Autodesk Inventor part; units mm, degrees
ref_plane "YZ Plane" through (0, 0, 0) normal (1, 0, 0) x (0, 1, 0)
ref_plane "XZ Plane" through (0, 0, 0) normal (0, 1, 0) x (-1, 0, 0)
ref_plane "XY Plane" through (0, 0, 0) normal (0, 0, 1) x (1, 0, 0)
sketch "Skizze1" plane through (0, 0, 0) normal (0, 0, 1) x (1, 0, 0)
  line L0 (-65.8319, 0) -> (313.5681, 0)
  line L1 (0, -176.4249) -> (0, 176.4249)
  line L2 (13.3681, -123) -> (13.3681, 123)
  line L3 (13.3681, -125.5) -> (259.3681, -125.5) construction
  line L4 (10.8681, 125.5) -> (-11.6319, 125.5)
  line L5 (-11.6319, 125.5) -> (-11.6319, 104.5)
  line L6 (10.8681, -125.5) -> (-11.6319, -125.5)
  line L7 (13.3681, -125.5) -> (35.8681, -125.5) construction
  line L8 (-11.6319, -125.5) -> (-11.6319, -124)
  line L9 (-11.6319, -124) -> (10.8681, -124)
  line L10 (11.8681, -123) -> (11.8681, 123)
  line L11 (10.8681, 124) -> (-10.1319, 124)
  line L12 (-10.1319, 124) -> (-10.1319, 104.5)
  line L13 (-10.1319, 104.5) -> (-11.6319, 104.5)
  arc A0 (13.3681, 123) -> (10.8681, 125.5) centre (10.8681, 123) ccw
  arc A1 (10.8681, -125.5) -> (13.3681, -123) centre (10.8681, -123) ccw
  arc A2 (10.8681, -124) -> (11.8681, -123) centre (10.8681, -123) ccw
  arc A3 (11.8681, 123) -> (10.8681, 124) centre (10.8681, 123) ccw
  point P0 (0, 0)
  point P1 (13.3681, 125.5)
  point P2 (11.8681, -124)
  point P3 (11.8681, 124)
  dimension "d0" = 251
  dimension "d1" = 90
  dimension "d2" = 25
  dimension "d3" = 90
  dimension "d4" = 21
  dimension "d5" = 90
  dimension "d6" = 25
  dimension "d7" = 180
  dimension "d8" = 1.5
  dimension "d9" = 90
  dimension "d10" = 23.5
  dimension "d11" = 90
  dimension "d12" = 248
  dimension "d13" = 90
  dimension "d14" = 22
  dimension "d15" = 90
  dimension "d17" = 1
extrude "Extrusion1" add sketch "Skizze1" along normal mid plane 193 contours L10 A3 L11 L1 L4 A0 L2 L0 | L0 L2 A1 L6 L1 L9 A2 L10 | L1 L6 L8 L9 | L11 L12 L13 L5 L4 L1
sketch "Skizze2" plane through (-11.6319, 104.5, 96.5) normal (-1, 0, 0) x (0, 0, 1)
  line L0 (-96.5, -280.2) -> (-96.5, 71.2)
  line L1 (-231.6, -104.5) -> (38.6, -104.5)
  line L2 (-193, 19.5) -> (-111.5, 19.5)
  line L3 (-111.5, 19.5) -> (-111.5, 0)
  line L4 (-111.5, 0) -> (-193, 0)
  line L5 (-193, 0) -> (-193, 19.5)
  line L6 (-193, -227.5) -> (-193, 18.5)
  line L7 (0, 21) -> (-193, 21)
  line L8 (0, 19.5) -> (-81.5, 19.5)
  line L9 (-81.5, 19.5) -> (-81.5, 0)
  line L10 (-81.5, 0) -> (0, 0)
  line L11 (0, 0) -> (0, 19.5)
  point P0 (-96.5, -104.5)
  dimension "d20" = 19.5
  dimension "d22" = 1.5
  dimension "d23" = 15
extrude "Extrusion2" cut sketch "Skizze2" against normal blind 2
sketch "Skizze3" plane through (-11.6319, 125.5, 96.5) normal (0, 1, 0) x (1, 0, 0)
  line L0 (-5, 96.5) -> (30, 96.5)
  line L1 (11.6319, 231.6) -> (11.6319, -38.6)
  line L2 (0, 0) -> (0, 81.5)
  line L3 (0, 81.5) -> (1.5, 81.5)
  line L4 (1.5, 81.5) -> (1.5, 0)
  line L5 (0, 81.5) -> (0, 0)
  line L6 (1.5, 0) -> (0, 0)
  line L7 (0, 0) -> (0, 193)
  line L8 (22.5, 0) -> (0, 0)
  line L9 (0, 193) -> (0, 111.5)
  line L10 (0, 111.5) -> (1.5, 111.5)
  line L11 (1.5, 111.5) -> (1.5, 193)
  line L12 (1.5, 193) -> (0, 193)
  point P0 (11.6319, 96.5)
  dimension "d27" = 1.5
  dimension "d28" = 15
extrude "Extrusion3" cut sketch "Skizze3" against normal blind 2 contours L7 L12 L11 L10 | L3 L4 L6 L2
fillet "Rundung1" radius 2.5 1 edges at (-11.6319, 125.5, 0)
fillet "Rundung2" radius 1 1 edges at (-10.1319, 124, 0)
hole "Bohrung1" at (-11.6319, 114.5, 0) direction (1, 0, 0) diameter 10 depth 8 tip angle 118
sketch "Skizze4" plane through (13.3681, -123, 96.5) normal (1, 0, 0) x (0, 0, -1)
  line L0 (231.6, 123) -> (-38.6, 123)
  line L1 (96.5, -52.7) -> (96.5, 298.7)
  line L2 (16, 203.5) -> (177, 203.5)
  line L3 (177, 203.5) -> (177, 128.5)
  line L4 (177, 128.5) -> (16, 128.5)
  line L5 (16, 128.5) -> (16, 203.5)
  line L6 (0, 0) -> (0, 246)
  line L7 (193, 0) -> (193, 246)
  line L8 (0, 248.5) -> (193, 248.5)
  point P0 (96.5, 123)
  dimension "d42" = 16
  dimension "d43" = 75
  dimension "d44" = 16
  dimension "d45" = 45
extrude "Extrusion4" cut sketch "Skizze4" against normal blind 2
hole "Bohrung2" at (13.3681, 83.5, -86.5) direction (-1, 0, 0) diameter 5 depth 8 tip angle 118
pattern_linear "Rechteckige Anordnung1" count 2 spacing 173 along (0, 0, 1) count 2 spacing 167 along (0, -1, 0) of "Bohrung2"
hole "Bohrung3" at (13.3681, -14.5, 29) direction (-1, 0, 0) diameter 2.5 depth 8 tip angle 118
pattern_linear "Rechteckige Anordnung2" count 2 spacing 58 along (0, 0, -1) count 2 spacing 49 along (0, -1, 0) of "Bohrung3"
sketch "Skizze5" plane through (13.3681, -123, 96.5) normal (1, 0, 0) x (0, 0, -1)
  line L0 (96.5, -52.7) -> (96.5, 298.7)
  line L1 (231.6, 123) -> (-38.6, 123)
  line L2 (20, -2.5) -> (20, 16)
  line L3 (25, -2.5) -> (25, 16)
  arc A0 (25, 16) -> (20, 16) centre (22.5, 16) ccw
  line L4 (0, 0) -> (0, 246)
  line L5 (0, -2.5) -> (193, -2.5)
  line L6 (20, -2.5) -> (25, -2.5)
  line L7 (173, -2.5) -> (173, 16)
  line L8 (168, -2.5) -> (168, 16)
  arc A1 (173, 16) -> (168, 16) centre (170.5, 16) ccw
  line L9 (173, -2.5) -> (168, -2.5)
  line L10 (20, 248.5) -> (20, 230)
  line L11 (25, 248.5) -> (25, 230)
  arc A2 (20, 230) -> (25, 230) centre (22.5, 230) ccw
  line L12 (20, 248.5) -> (25, 248.5)
  line L13 (173, 248.5) -> (173, 230)
  arc A3 (168, 230) -> (173, 230) centre (170.5, 230) ccw
  line L14 (168, 248.5) -> (168, 230)
  line L15 (173, 248.5) -> (168, 248.5)
  point P0 (96.5, 123)
  point P1 (0, 248.5)
  point P2 (193, 248.5)
  dimension "d78" = 5
  dimension "d79" = 22.5
  dimension "d80" = 18.5
extrude "Extrusion5" cut sketch "Skizze5" against normal blind 5
sketch "Skizze6" plane through (-9.1319, 125.5, -96.5) normal (0, 1, 0) x (1, 0, 0)
  line L0 (9.1319, 38.6) -> (9.1319, -231.6)
  line L1 (-7.5, -96.5) -> (27.5, -96.5)
  line L2 (7.5, -173) -> (20.5, -173)
  line L3 (21, -177) -> (21, -16)
  line L4 (20.5, -173) -> (20.5, -168)
  line L5 (20.5, -168) -> (7.5, -168)
  line L6 (22.5, -193) -> (22.5, -173)
  line L7 (17.5, -168) -> (20, -168)
  arc A0 (7.5, -168) -> (7.5, -173) centre (7.5, -170.5) ccw
  line L8 (7.5, -20) -> (20.5, -20)
  line L9 (20.5, -20) -> (20.5, -25)
  line L10 (20.5, -25) -> (7.5, -25)
  line L11 (17.5, -25) -> (20, -25)
  arc A1 (7.5, -20) -> (7.5, -25) centre (7.5, -22.5) ccw
  point P0 (9.1319, -96.5)
  dimension "d83" = 5
  dimension "d84" = 2
  dimension "d85" = 15
extrude "Extrusion6" cut sketch "Skizze6" against normal through all
fillet "Rundung3" radius 5 4 edges at (12.6181, 5.5, 80.5) (12.6181, 80.5, 80.5) (12.6181, 80.5, -80.5) (12.6181, 5.5, -80.5)
fillet "Rundung4" radius 5 4 edges at (-10.1319, 124.6456, -96.5) (-11.6319, -124.75, -96.5) (-11.6319, -124.75, 96.5) (-10.1319, 124.6456, 96.5)
properties part number "Innengehäuse gebogen" material "Stahl AISI 1015"
Verification items for the finished model (mm, model axes). A direction names the side the tool comes from. Round coordinates to 2 decimals unless told otherwise and drop trailing zeros. Write each loop counter-clockwise with the first axis right and the second up, starting at its lowest first coordinate (ties: lowest second). Pieces come first, ordered by that corner, then holes. Notation, with made-up numbers: (5, 50.25) - (34, 50.25) arc R18 ccw to (34, 81.25) - close; hole circle Ø1 at (-16.75, 69.5). An arc over 180 degrees is marked (long way). Answer as a JSON object with one key per item and string values. Group by question number.
Q1. Go/stop test with flat-tipped pins: pin 1 Ø1 at (y, z) = (125, -49.5) entering from -X; pin 2 Ø2 at (y, z) = (-63.5, -29) entering from +X; pin 3 Ø0.8 at (x, y) = (-10.5, 115) entering from -Z; pin 4 Ø9 at (y, z) = (114.5, 0) entering from -X. Record where each tip stops, or that it passes through.
Q2. Thickness scan on line 1 (Z direction, x = 12.6, y = 83.5); line 2 (Z direction, x = 12.5, y = -63.5); line 3 (Y direction, x = 8.5, z = -41). Record the ranges inside material, lowest first.
Q3. Mould release check, pull along Z, two halves, no side actions. Record for faces 1 (the flat face through (13, -118, 76.5)), 2 (the flat face through (1, 124, -1)), 3 (the flat face through (12.2, 0.6, -96.5)): released by +Z, released by -Z, zero draft, split by the parting line, or undercut.
Q4. Section check D-D, the plane y = -38.5. Enter the section's corners in (x, z), plus the area to 4 significant figures.
Q5. Section check B-B, the plane x = 4.5. Enter the section's corners in (y, z).
Q6. Section check A-A, the plane z = -23.5. Enter the section's corners in (x, y), plus the area to 3 significant figures.
Q7. Section check C-C, the plane z = 0. Enter the section's corners in (x, y).
Q8. Tool access check on faces 4 (the cylindrical face through (12.61, 79.07, -79)), 5 (the flat face through (13, 118, 76.5)), 6 (the cylindrical face through (-10.871, 110.284, 2.688)), 7 (the flat face through (13, -118, -76.5)), 8 (the cylindrical face through (-8.6, 124.7, 95.1)). Record the directions out of +Z, -Z, +X, -X, +Y, -Y that give a thin tool (end or side, any length) a straight path to the whole face; none if there is none.
Found:
{
 "1": {"pin 1": "stops at x = -10.13", "pin 2": "passes through", "pin 3": "stops at z = -15", "pin 4": "stops at x = 11.87"},
 "2": {"line 1": "z = -96.5 to -89, -84 to 84, 89 to 96.5", "line 2": "z = -96.5 to -30.25, -27.75 to 27.75, 30.25 to 96.5", "line 3": "y = -125.5 to -124, 124 to 125.5"},
 "3": {"face 1": "undercut", "face 2": "zero draft", "face 3": "released by -Z"},
 "4": {"outline": "(11.87, -96.5) - (13.37, -96.5) - (13.37, 96.5) - (11.87, 96.5) - close", "area": "289.5 mm^2"},
 "5": {"outline": "(-125.5, -96.5) - (-124, -96.5) - (-124, -76.5) - (-125.5, -76.5) - close; (-125.5, -71.5) - (-124, -71.5) - (-124, 71.5) - (-125.5, 71.5) - close; (-125.5, 76.5) - (-124, 76.5) - (-124, 96.5) - (-125.5, 96.5) - close; (124, -96.5) - (125.5, -96.5) - (125.5, -76.5) - (124, -76.5) - close; (124, -71.5) - (125.5, -71.5) - (125.5, 71.5) - (124, 71.5) - close; (124, 76.5) - (125.5, 76.5) - (125.5, 96.5) - (124, 96.5) - close"},
 "6": {"outline": "(-11.63, -125.5) - (10.87, -125.5) arc R2.5 ccw to (13.37, -123) - (13.37, 5.5) - (11.87, 5.5) - (11.87, -123) arc R1 cw to (10.87, -124) - (-11.63, -124) - close; (-10.13, 124) - (10.87, 124) arc R1 cw to (11.87, 123) - (11.87, 80.5) - (13.37, 80.5) - (13.37, 123) arc R2.5 ccw to (10.87, 125.5) - (-9.13, 125.5) arc R2.5 ccw to (-10.13, 125.29) - close", "area": "330 mm^2"},
 "7": {"outline": "(-11.63, -125.5) - (10.87, -125.5) arc R2.5 ccw to (13.37, -123) - (13.37, 5.5) - (11.87, 5.5) - (11.87, -123) arc R1 cw to (10.87, -124) - (-11.63, -124) - close; (-11.63, 104.5) - (-10.13, 104.5) - (-10.13, 109.5) - (-11.63, 109.5) - close; (-11.63, 119.5) - (-10.13, 119.5) - (-10.13, 123) arc R1 cw to (-9.13, 124) - (10.87, 124) arc R1 cw to (11.87, 123) - (11.87, 80.5) - (13.37, 80.5) - (13.37, 123) arc R2.5 ccw to (10.87, 125.5) - (-9.13, 125.5) arc R2.5 ccw to (-11.63, 123) - close"},
 "8": {"face 4": "+X, -X", "face 5": "+X, +Y", "face 6": "-X", "face 7": "+X, -Y", "face 8": "+Z, -X, +Y"}
}
